```python
from build123d import *

# Parameters (mm, degrees)
F0_W     = 76.2
F0_H     = 76.2
F1_DEPTH = 76.2
F2_W     = 31.75
F2_H     = 31.75
F3_DEPTH = 102.87
F4_DEPTH = 134.874
F5_DEPTH = 137.922
F6_DEPTH = 121.412
F7_W     = 31.75
F7_H     = 31.75
F8_DEPTH = 107.696


with BuildPart() as f1:
    # F0 (on Top) → F1 (new body)
    with BuildSketch(Plane.XY):
        Rectangle(F0_W, F0_H)
    extrude(amount=F1_DEPTH)

    # F2 (on face) → F3 (cut)
    with BuildSketch(Plane.XY.offset(76.2)):
        with Locations((-19.05, 19.05)):
            Rectangle(F2_W, F2_H)
    extrude(amount=-F3_DEPTH, mode=Mode.SUBTRACT)

    # F2 (on face) → F4 (cut)
    with BuildSketch(Plane.XY.offset(76.2)):
        with Locations((19.05, 19.05)):
            Rectangle(F2_W, F2_H)
    extrude(amount=-F4_DEPTH, mode=Mode.SUBTRACT)

    # F2 (on face) → F5 (cut)
    with BuildSketch(Plane.XY.offset(76.2)):
        with Locations((-19.05, -19.05)):
            Rectangle(F2_W, F2_H)
    extrude(amount=-F5_DEPTH, mode=Mode.SUBTRACT)

    # F2 (on face) → F6 (cut)
    with BuildSketch(Plane.XY.offset(76.2)):
        with Locations((19.05, -19.05)):
            Rectangle(F2_W, F2_H)
    extrude(amount=-F6_DEPTH, mode=Mode.SUBTRACT)

    # F7 (on face) → F8 (cut)
    with BuildSketch(Plane.YZ.offset(38.1)):
        with Locations((-19.05, 57.15)):
            Rectangle(F7_W, F7_H)
        with Locations((19.05, 57.15)):
            Rectangle(F7_W, F7_H)
        with Locations((-19.05, 19.05)):
            Rectangle(F7_W, F7_H)
        with Locations((19.05, 19.05)):
            Rectangle(F7_W, F7_H)
    extrude(amount=-F8_DEPTH, mode=Mode.SUBTRACT)


solid = f1.part
```
Geometry: final body of the model. Coordinates: model frame, mm. A direction names the side the tool comes from. Coordinates: 2 decimals unless noted, no trailing zeros. Loops run counter-clockwise (first coordinate to the right, second up) from the corner with the lowest first, then second, coordinate; pieces in that order, holes last. Notation, with made-up numbers: (19.5, -30) -> (72.5, -30) arc R26 ccw to (72.5, -4) -> close; hole circle Ø10 at (-40, 59). An arc over 180 degrees is marked (long way). Use a Markdown table: item, result. Add a question column.
(1) Mould query, pull axis Z, two halves, no side actions, for faces 1 (the flat face through (-3, 0, 0)), 2 (the flat face through (34.925, 19, 38)), 3 (the flat face through (-36, 19, 41.275)). Classes: pulls with the +Z half, pulls with the -Z half, needs draft (parallel to the pull), parting line crosses it, or undercut.
(2) Line query: line 1 along Y through (x, z) = (-5.5, 56) (3 decimals); line 2 along Z through (x, y) = (-2, 6.5) (3 decimals). Output: solid intervals per line, ascending.
(3) Access query for faces 4 (the flat face through (-36, 19, 34.925)), 5 (the flat face through (3.175, -19, 75)). Directions: +Z, -Z, +X, -X, +Y, -Y. A direction counts if a zero-diameter tool reaches every point of the face in a straight line with its end or side. Return the directions, or none.
(4) Section query B-B, the plane z = 26. Return loops of the section in (x, y) (3 decimals), plus the area to 3 significant figures.
(5) Section query A-A, the plane x = 7.5. Return loops of the section in (y, z) (3 decimals), plus the area to 3 significant figures.
(6) Section query C-C, the plane y = -19. State how many separate pieces and enclosed holes the cut face has, plus the area to 3 significant figures.
(7) Pin query (flat end, axial travel): pin 1 Ø6 at (x, y) = (-8.5, 21.5) entering from -Z. Return the tip coordinate at first contact, or that it passes through.
Answer:
| question | item | result |
|---|---|---|
| 1 | face 1 | pulls with the -Z half |
| 1 | face 2 | needs draft |
| 1 | face 3 | undercut |
| 2 | line 1 | y = -38.1 to -34.925, -3.175 to 3.175, 34.925 to 38.1 |
| 2 | line 2 | z = 0 to 3.175, 34.925 to 41.275, 73.025 to 76.2 |
| 3 | face 4 | +X, -X |
| 3 | face 5 | +Z, -Z |
| 4 | outline | (-38.1, -38.1) -> (38.1, -38.1) -> (38.1, -34.925) -> (-38.1, -34.925) -> close; (-38.1, -3.175) -> (38.1, -3.175) -> (38.1, 3.175) -> (-38.1, 3.175) -> close; (-38.1, 34.925) -> (38.1, 34.925) -> (38.1, 38.1) -> (-38.1, 38.1) -> close |
| 4 | area | 968 mm^2 |
| 5 | outline | (-38.1, 0) -> (-34.925, 0) -> (-34.925, 76.2) -> (-38.1, 76.2) -> close; (-3.175, 0) -> (3.175, 0) -> (3.175, 76.2) -> (-3.175, 76.2) -> close; (34.925, 0) -> (38.1, 0) -> (38.1, 76.2) -> (34.925, 76.2) -> close |
| 5 | area | 968 mm^2 |
| 6 | separate pieces | 9 |
| 6 | enclosed holes | 0 |
| 6 | area | 161 mm^2 |
| 7 | pin 1 | passes through |
